Work out the finished part from the listing and answer in its coordinate system (mm). Face numbers are marked on the shaded views. A direction names the side the tool comes from. Coordinates: 2 decimals unless noted, no trailing zeros. Write each loop counter-clockwise with the first axis right and the second up, starting at its lowest first coordinate (ties: lowest second). Pieces come first, ordered by that corner, then holes. Notation, with made-up numbers: (-7, -28) - (45, -28) arc R18 cw to (45, -3) - close; hole circle Ø2 at (-32, 34.25). An arc over 180 degrees is marked (long way). Use CSV: the item, a comma, the result in double quotes. Start each with the question number.
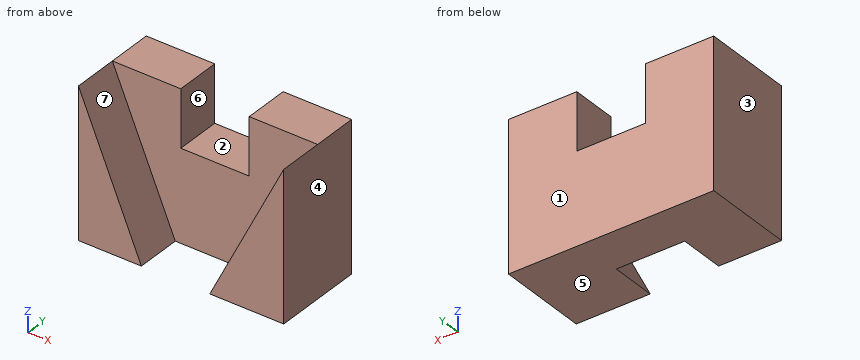
from build123d import *

# Parameters (mm, degrees)
F0_W     = 90
F0_H     = 65
F1_DEPTH = 40
F3_DEPTH = 20
F4_W     = 30
F4_H     = 50
F5_DEPTH = 20.001


with BuildPart() as f1:
    # F0 (on Front) → F1 (new body)
    with BuildSketch(Plane.XZ):
        Rectangle(F0_W, F0_H)
    extrude(amount=F1_DEPTH)

    # F2 (on face) → F3 (cut)
    with BuildSketch(Plane.XZ.offset(40)):
        Polygon((-45, 32.5), (-17.421313, -32.5), (12.578687, -32.5), (45, 32.5), align=None)
    extrude(amount=-F3_DEPTH, mode=Mode.SUBTRACT)

    # F4 (on face) → F5 (cut, through all)
    with BuildSketch(Plane.XZ.offset(20)):
        with Locations((0, 32.5)):
            Rectangle(F4_W, F4_H)
    extrude(amount=-F5_DEPTH, mode=Mode.SUBTRACT)


solid = f1.part
Item 1: Straight lines are drawn through the part: probe 1 along X at (y, z) = (-2.5, 9); probe 2 along Y at (x, z) = (-19.5, -27.5); probe 3 along Z at (x, y) = (12, -9.5). For each, find the intervals that lie inside material, in ascending order. Write a range as [from, to].
Item 2: A cutting plane is placed at A-A (y = -23.5). Determine the outline of the cut face in (x, z), then the cut area to 3 significant figures.
Item 3: A cutting plane is placed at C-C (z = 10). Determine the outline of the cut face in (x, y).
Item 4: A cutting plane is placed at D-D (x = 22). Determine the outline of the cut face in (y, z).
Item 5: Determine the mould class of the marked faces 1, 2, 3 and 4 for opening direction X: +X half, -X half, draft (parallel to the pull), parting line (faces both ways), or undercut.
Item 6: A cutting plane is placed at B-B (y = -8.5). Determine the outline of the cut face in (x, z).
Item 7: Which of the six approach directions +Z, -Z, +X, -X, +Y, -Y give full straight-line access (tool end or side, diameter ignored) to the marked faces 5, 6 and 7?
Item 8: Each of these flat-tipped pins is pushed along its axis until it touches: pin 1 (12 mm diameter, centred on x = 3.5, y = -27, fed in from -Z); pin 2 (19.5 mm diameter, centred on x = -18, z = 14.5, fed in from -Y); pin 3 (2 mm diameter, centred on x = 22, y = -31.5, fed in from +Z); pin 4 (10 mm diameter, centred on x = 5.5, y = -10, fed in from +Z). Where does it stop, or does it pass through?
Calculated:
1,probe 1,"x = [-45, -15], [15, 45]"
1,probe 2,"y = [-20, 0]"
1,probe 3,"z = [-32.5, 7.5]"
2,outline,"(-45, -32.5) - (-17.42, -32.5) - (-45, 32.5) - close; (12.58, -32.5) - (45, -32.5) - (45, 32.5) - close"
2,area,"1,950 mm²"
3,outline,"(-45, -40) - (-35.45, -40) - (-35.45, -20) - (-15, -20) - (-15, 0) - (-45, 0) - close; (15, -20) - (33.78, -20) - (33.78, -40) - (45, -40) - (45, 0) - (15, 0) - close"
4,outline,"(-40, -32.5) - (0, -32.5) - (0, 32.5) - (-20, 32.5) - (-20, -13.61) - (-40, -13.61) - close"
5,face 1,"draft"
5,face 2,"undercut"
5,face 3,"-X half"
5,face 4,"+X half"
6,outline,"(-45, -32.5) - (45, -32.5) - (45, 32.5) - (15, 32.5) - (15, 7.5) - (-15, 7.5) - (-15, 32.5) - (-45, 32.5) - close"
7,face 5,"-Z, +X, -X, +Y, -Y"
7,face 6,"+Z, +Y, -Y"
7,face 7,"+Z, -Y"
8,pin 1,"passes through"
8,pin 2,"stops at y = -20"
8,pin 3,"stops at z = -11.61"
8,pin 4,"stops at z = 7.5"
